```python
from build123d import *

# Parameters (mm, degrees)
F0_W     = 1000
F0_H     = 330
F1_DEPTH = 180
F0_H_2   = 540
F2_DEPTH = 335
F3_W     = 190
F3_H     = 130
F4_DEPTH = 1000
F6_DEPTH = 1000


with BuildPart() as f1:
    # F0 (on Top) → F1 (new body)
    with BuildSketch(Plane.XY):
        with Locations((500, -705)):
            Rectangle(F0_W, F0_H)
    extrude(amount=F1_DEPTH)

    # F0 (on Top) → F2 (join)
    with BuildSketch(Plane.XY):
        with Locations((500, -270)):
            Rectangle(F0_W, F0_H_2)
    extrude(amount=F2_DEPTH)

    # F3 (on face) → F4 (join)
    with BuildSketch(Plane.YZ.offset(1000)):
        with Locations((-95, 230)):
            Rectangle(F3_W, F3_H)
    extrude(amount=F4_DEPTH)

    # F3 (on face) → F6 (join)
    with BuildSketch(Plane.YZ.offset(1000)):
        with Locations((-95, 230)):
            Rectangle(F3_W, F3_H)
        with BuildLine():
            Line((-870, 50), (-870, 0))
            Line((-870, 0), (-770, 0))
            Line((-770, 0), (-770, 80))
            Line((-770, 80), (-840, 80))
            ThreePointArc((-840, 80), (-861.213203, 71.213203), (-870, 50))
        make_face()
    extrude(amount=F6_DEPTH)


solid = f1.part
```
Model file for the job. Use its own axes, mm. A direction names the side the tool comes from. Coordinates: 2 decimals unless noted, no trailing zeros. Order: outer loops, then holes, each group sorted by start corner. A loop starts at its lowest first (then second) coordinate and runs counter-clockwise, first axis right, second up. Notation, with made-up numbers: (-15, 3) - (34, 3) arc R6 ccw to (34, 14) - close; hole circle Ø8 at (25, 33.5). An arc over 180 degrees is marked (long way). Return JSON: item names as keys, results as strings. Group by question number.
1) Flat gauge pins, fed straight in: P1, Ø3, axis at x = 1537.5, y = -181.5, coming from the +Z side; P2, Ø4, axis at y = -420.5, z = 210.5, coming from the +X side; P3, Ø5, axis at y = -633.5, z = 144, coming from the -X side; P4, Ø3, axis at x = 903.5, z = 267.5, coming from the -Y side. Where does each tip first touch, or does it go through?
2) Probe line 1 (X direction, y = -540, z = 66); line 2 (Y direction, x = 1694.5, z = 280); line 3 (Z direction, x = 255, y = -679.5). List the from-to ranges inside material, lowest first. Write a range as from..to.
3) Saw through at A-A, the plane y = -85. Write the cut outline in (x, z), plus the area to 3 significant figures.
4) Saw through at C-C, the plane z = 218.5. Write the cut outline in (x, y).
5) Saw through at B-B, the plane x = 1693.5. Write the cut outline in (y, z).
6) Saw through at D-D, the plane x = 823.5. Write the cut outline in (y, z).
7) Tool access for faces 1 (the flat face through (493, -540, 256)), 2 (the flat face through (1493, -96, 165)), 3 (the flat face through (1493, -190, 229)), 4 (the flat face through (1493, -805, 80)), 5 (the flat face through (1493, -770, 39)): list every direction of +Z, -Z, +X, -X, +Y, -Y with a clear straight run to the whole face (end or side of a thin tool).
Values found:
{
 "1": {"P1": "stops at z = 295", "P2": "stops at x = 1000", "P3": "stops at x = 0", "P4": "stops at y = -540"},
 "2": {"line 1": "x = 0..1000", "line 2": "y = -190..0", "line 3": "z = 0..180"},
 "3": {"outline": "(0, 0) - (1000, 0) - (1000, 165) - (2000, 165) - (2000, 295) - (1000, 295) - (1000, 335) - (0, 335) - close", "area": "465,000 mm²"},
 "4": {"outline": "(0, -540) - (1000, -540) - (1000, -190) - (2000, -190) - (2000, 0) - (0, 0) - close"},
 "5": {"outline": "(-870, 0) - (-770, 0) - (-770, 80) - (-840, 80) arc R30 ccw to (-870, 50) - close; (-190, 165) - (0, 165) - (0, 295) - (-190, 295) - close"},
 "6": {"outline": "(-870, 0) - (0, 0) - (0, 335) - (-540, 335) - (-540, 180) - (-870, 180) - close"},
 "7": {"face 1": "+Z, +X, -X, -Y", "face 2": "-Z, +X, +Y, -Y", "face 3": "+Z, -Z, +X, -Y", "face 4": "+Z, +X, +Y, -Y", "face 5": "+Z, -Z, +X, +Y"}
}
